Source: CAD feature listing. Evaluate the final solid. Frame: model axes, mm. A direction names the side the tool comes from. Coordinates: 2 decimals unless noted, no trailing zeros. Loops run counter-clockwise (first coordinate to the right, second up) from the corner with the lowest first, then second, coordinate; pieces in that order, holes last.
Item 1: Line query: probe 1 along X at (y, z) = (-3.75, 7.25); probe 2 along Y at (x, z) = (2.5, -3.25); probe 3 along X at (y, z) = (-3, -7.5). Output: solid intervals per line, ascending.
Item 2: Reachability of faces 5 (the flat face through (14, -5, -5)), 6 (the flat face through (-5.7, -4, -7)), 7 (the flat face through (-4, -4, -5.2)), 8 (the flat face through (-8.75, 1, -4)), 9 (the flat face through (-2.8, -4, -7)) from +Z, -Z, +X, -X, +Y, -Y: full face, straight path, thin tool, end or side. Return the list, or none.
Item 3: Section query B-B, the plane z = -4.8. Return the cut outline in (x, y), then the cut area to 3 significant figures.
Item 4: Section query D-D, the plane y = -5.5. Return the cut outline in (x, z), then the cut area to 3 significant figures.
Item 5: Section query C-C, the plane x = -13. Return the cut outline in (y, z), then the cut area to 3 significant figures.
Item 6: Section query A-A, the plane y = -2.5. Return the cut outline in (x, z), then the cut area to 3 significant figures.
Item 7: Pull-direction query (Z, two-part tool) for faces 1 (the flat face through (0.5, 0.3, -8)), 2 (the flat face through (-4, -8, -7)), 3 (the flat face through (11, -2, 6.9)), 4 (the flat face through (0, 1, 8)); classes: +Z half, -Z half, draft (parallel to the pull), parting line (faces both ways), or undercut.
Item 8: Pin query (flat end, axial travel): pin 1 Ø1.2 at (x, z) = (-12, 7.5) entering from -Y; pin 2 Ø1.4 at (y, z) = (-5.5, -6.5) entering from +X; pin 3 Ø5 at (x, z) = (2, 1) entering from -Y. Return the tip coordinate at first contact, or that it passes through.
```python
from build123d import *

# Parameters (mm, degrees)
SKETCH1_W           = 30.5
SKETCH1_H           = 16
BOSS_EXTRUDE1_DEPTH = 2
SKETCH3_R           = 1
SKETCH3_W           = 2.9
SKETCH3_H           = 2.8
SKETCH3_W_2         = 8
SKETCH3_H_2         = 1.1
BOSS_EXTRUDE3_DEPTH = 8
CUT_EXTRUDE2_DEPTH  = 10
CUT_EXTRUDE3_START  = -3
SKETCH5_R           = 1
SKETCH5_W           = 30.5
SKETCH5_H           = 1.1
CUT_EXTRUDE3_DEPTH  = 3


with BuildPart() as part:
    # Sketch1 → Boss-Extrude1 (new body)
    with BuildSketch(Plane(origin=(0, 0, 0), x_dir=(1, 0, 0), z_dir=(0, 1, 0))):
        Rectangle(SKETCH1_W, SKETCH1_H)
    extrude(amount=BOSS_EXTRUDE1_DEPTH)

    # Sketch3 → Boss-Extrude3 (add)
    with BuildSketch(Plane(origin=(0, 0, 0), x_dir=(1, 0, 0), z_dir=(0, 1, 0))):
        with Locations(Location((14.2, 4.8, 0), (0, 0, 270))):
            Circle(SKETCH3_R)
        with Locations((-4.25, 6.6)):
            Rectangle(SKETCH3_W, SKETCH3_H)
        with Locations((-11.25, -7.45)):
            Rectangle(SKETCH3_W_2, SKETCH3_H_2)
        with Locations((11.25, -7.45)):
            Rectangle(SKETCH3_W_2, SKETCH3_H_2)
    extrude(amount=-BOSS_EXTRUDE3_DEPTH)

    # Sketch4 → Cut-Extrude2 (cut)
    with BuildSketch(Plane(origin=(0, 0, 0), x_dir=(1, 0, 0), z_dir=(0, 1, 0))):
        Polygon((-15.25, 2.7), (-15.25, 8), (-8.75, 8), (-8.75, 2.7), (-8.75, 0.2), (-15.25, 0.2), align=None)
    extrude(amount=CUT_EXTRUDE2_DEPTH, mode=Mode.SUBTRACT)

    # Sketch5 → Cut-Extrude3 (cut)
    with BuildSketch(Plane.XZ.offset(8).offset(CUT_EXTRUDE3_START)):
        with Locations(Location((14.2, -4.8, 0), (0, 0, 90))):
            Circle(SKETCH5_R)
        with Locations((0, 7.45)):
            Rectangle(SKETCH5_W, SKETCH5_H)
    extrude(amount=CUT_EXTRUDE3_DEPTH, mode=Mode.SUBTRACT)


solid = part.part
```
Verdict:
1. probe 1: x = -15.25 to -7.25, 7.25 to 15.25
1. probe 2: y = 0 to 2
1. probe 3: x = -5.7 to -2.8
2. face 5: +Z, -Z, +X, -Y
2. face 6: +Z, -Z, -X, -Y
2. face 7: +Z, -X, -Y
2. face 8: -Z, -X, +Y, -Y
2. face 9: +Z, -Z, -Y
3. outline: (-8.75, 0) - (13.2, 0) - (13.2, -5) - (15.2, -5) - (15.2, 0) - (15.25, 0) - (15.25, 2) - (-8.75, 2) - close
3. area: 58.0 mm2
4. outline: (-5.7, -8) - (-2.8, -8) - (-2.8, -5.2) - (-5.7, -5.2) - close
4. area: 8.12 mm2
5. outline: (-5, 6.9) - (0, 6.9) - (0, -0.2) - (2, -0.2) - (2, 8) - (-5, 8) - close
5. area: 21.9 mm2
6. outline: (-15.25, 6.9) - (-7.25, 6.9) - (-7.25, 8) - (-15.25, 8) - close; (-5.7, -8) - (-2.8, -8) - (-2.8, -5.2) - (-5.7, -5.2) - close; (7.25, 6.9) - (15.25, 6.9) - (15.25, 8) - (7.25, 8) - close; circle Ø2 at (14.2, -4.8)
6. area: 28.9 mm2
7. face 1: -Z half
7. face 2: draft
7. face 3: undercut
7. face 4: +Z half
8. pin 1: stops at y = -5
8. pin 2: stops at x = -2.8
8. pin 3: stops at y = 0
